Verification items for the finished model (mm, model axes). Face numbers are marked on the shaded views. A direction names the side the tool comes from. Give positions to 0.01 mm unless a question says otherwise; leave off trailing zeros. Order: outer loops, then holes, each group sorted by start corner. A loop starts at its lowest first (then second) coordinate and runs counter-clockwise, first axis right, second up. Notation, with made-up numbers: (19.5, 33) -> (61.5, 33) arc R26 cw to (61.5, 61) -> close; hole circle Ø5 at (33.5, -16). An arc over 180 degrees is marked (long way). Write each question's results on one line, items separated by ' | '. Start each with the question number.
1. Material ranges on L1, parallel to Y at x = -15, z = 28; L2, parallel to Z at x = -14, y = -24; L3, parallel to Z at x = 10, y = 3.45, recorded low to high. Write a range as from..to.
2. Cross-section at C-C, the plane y = -6. State how many separate pieces and enclosed holes the cut face has, then the cut area to 3 significant figures.
3. Mould release check, pull along Z, two halves, no side actions. Record for the marked faces 5, 6 and 7: +Z half, -Z half, draft (parallel to the pull), parting line (faces both ways), or undercut.
4. Cross-section at D-D, the plane x = -11.5. Enter the section's corners in (y, z), then the cut area to 3 significant figures.
5. Cross-section at A-A, the plane x = 10. Enter the section's corners in (y, z).
6. Cross-section at B-B, the plane z = 18. Enter the section's corners in (x, y).
7. Set-up check for the marked faces 1, 2, 3 and 4: record each of +Z, -Z, +X, -X, +Y, -Y from which the full face is reachable in a straight line by a thin tool's end or side.
8. Depth check by flat-ended pin: pin 1 Ø9 at (y, z) = (-25.5, 25.5) entering from -X; pin 2 Ø5 at (y, z) = (-24, 47) entering from +X; pin 3 Ø7 at (y, z) = (-6, 28) entering from +X; pin 4 Ø12 at (y, z) = (-23.5, 47.5) entering from -X. Enter the tip coordinate at first touch or a pass-through.
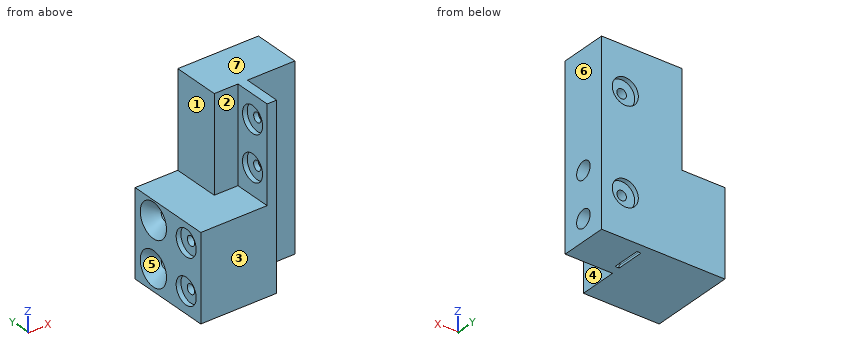
from build123d import *

# Parameters (mm, degrees)
CYLINDER007_R     = 5.5
CYLINDER007_DEPTH = 2
CYLINDER001_R     = 2
CYLINDER001_DEPTH = 32
CYLINDER006_R     = 5.5
CYLINDER006_DEPTH = 2
CYLINDER_R        = 2
CYLINDER_DEPTH    = 32
CYLINDER011_R     = 2
CYLINDER011_DEPTH = 20
CYLINDER013_R     = 5.5
CYLINDER013_DEPTH = 2
CYLINDER008_R     = 5.5
CYLINDER008_DEPTH = 2
CYLINDER002_R     = 2
CYLINDER002_DEPTH = 4
CYLINDER012_R     = 2
CYLINDER012_DEPTH = 20
CYLINDER010_R     = 5.5
CYLINDER010_DEPTH = 2
CYLINDER009_R     = 5.5
CYLINDER009_DEPTH = 2
CYLINDER003_R     = 2
CYLINDER003_DEPTH = 4
CYLINDER004_R     = 2.2
CYLINDER004_DEPTH = 22
CYLINDER015_R     = 3.7
CYLINDER015_DEPTH = 30
CYLINDER014_R     = 3.7
CYLINDER014_DEPTH = 30
CYLINDER005_R     = 2.2
CYLINDER005_DEPTH = 22
BOX002_W          = 20
BOX002_H          = 4
BOX002_DEPTH      = 76
BOX005_W          = 20
BOX005_H          = 12
BOX005_DEPTH      = 40
BOX011_W          = 18
BOX011_H          = 12
BOX011_DEPTH      = 36
BOX009_W          = 0.3
BOX009_H          = 12
BOX009_DEPTH      = 1
BOX_W             = 20
BOX_H             = 4
BOX_DEPTH         = 76
BOX012_W          = 10
BOX012_H          = 20
BOX012_DEPTH      = 40
BOX010_W          = 28
BOX010_H          = 36
BOX010_DEPTH      = 36
BOX001_W          = 4
BOX001_H          = 36
BOX001_DEPTH      = 76
CHAMFER_SIZE      = 5


with BuildPart() as cylinder007:
    # Cylinder007 → Cylinder007 (new body)
    with BuildSketch(Plane(origin=(-24, -24, 28), x_dir=(0, 0, -1), z_dir=(1, 0, 0))):
        Circle(CYLINDER007_R)
    extrude(amount=CYLINDER007_DEPTH)


with BuildPart() as fusion:
    # Cylinder001 → Cylinder001 (new body)
    with BuildSketch(Plane(origin=(-24, -24, 28), x_dir=(0, 0, -1), z_dir=(1, 0, 0))):
        Circle(CYLINDER001_R)
    extrude(amount=CYLINDER001_DEPTH)

    # Fusion: union Cylinder007
    add(cylinder007.part)


with BuildPart() as fusion_1:
    # Fusion placement: moved
    add(fusion.part.moved(Location((-8, 0, 0))))


with BuildPart() as cylinder006:
    # Cylinder006 → Cylinder006 (new body)
    with BuildSketch(Plane(origin=(-24, -24, 9), x_dir=(0, 0, -1), z_dir=(1, 0, 0))):
        Circle(CYLINDER006_R)
    extrude(amount=CYLINDER006_DEPTH)


with BuildPart() as fusion005:
    # Cylinder → Cylinder (new body)
    with BuildSketch(Plane(origin=(-24, -24, 9), x_dir=(0, 0, -1), z_dir=(1, 0, 0))):
        Circle(CYLINDER_R)
    extrude(amount=CYLINDER_DEPTH)

    # Fusion005: union Cylinder006
    add(cylinder006.part)


with BuildPart() as fusion005_1:
    # Fusion005 placement: moved
    add(fusion005.part.moved(Location((-8, 0, 0))))


with BuildPart() as cylinder011:
    # Cylinder011 → Cylinder011 (new body)
    with BuildSketch(Plane(origin=(10, 4, 58), x_dir=(1, 0, 0), z_dir=(0, -1, 0))):
        Circle(CYLINDER011_R)
    extrude(amount=CYLINDER011_DEPTH)


with BuildPart() as fusion012:
    # Cylinder013 → Cylinder013 (new body)
    with BuildSketch(Plane(origin=(10, 4, 58), x_dir=(1, 0, 0), z_dir=(0, -1, 0))):
        Circle(CYLINDER013_R)
    extrude(amount=CYLINDER013_DEPTH)

    # Fusion012: union Cylinder011
    add(cylinder011.part)


with BuildPart() as cylinder008:
    # Cylinder008 → Cylinder008 (new body)
    with BuildSketch(Plane(origin=(-4, -24, 47), x_dir=(0, 0, -1), z_dir=(1, 0, 0))):
        Circle(CYLINDER008_R)
    extrude(amount=CYLINDER008_DEPTH)


with BuildPart() as fusion007:
    # Cylinder002 → Cylinder002 (new body)
    with BuildSketch(Plane(origin=(-4, -24, 47), x_dir=(0, 0, -1), z_dir=(1, 0, 0))):
        Circle(CYLINDER002_R)
    extrude(amount=CYLINDER002_DEPTH)

    # Fusion007: union Cylinder008
    add(cylinder008.part)


with BuildPart() as cylinder012:
    # Cylinder012 → Cylinder012 (new body)
    with BuildSketch(Plane(origin=(10, 4, 18), x_dir=(1, 0, 0), z_dir=(0, -1, 0))):
        Circle(CYLINDER012_R)
    extrude(amount=CYLINDER012_DEPTH)


with BuildPart() as fusion011:
    # Cylinder010 → Cylinder010 (new body)
    with BuildSketch(Plane(origin=(10, 4, 18), x_dir=(1, 0, 0), z_dir=(0, -1, 0))):
        Circle(CYLINDER010_R)
    extrude(amount=CYLINDER010_DEPTH)

    # Fusion011: union Cylinder012
    add(cylinder012.part)


with BuildPart() as cylinder009:
    # Cylinder009 → Cylinder009 (new body)
    with BuildSketch(Plane(origin=(-4, -24, 66), x_dir=(0, 0, -1), z_dir=(1, 0, 0))):
        Circle(CYLINDER009_R)
    extrude(amount=CYLINDER009_DEPTH)


with BuildPart() as fusion006:
    # Cylinder003 → Cylinder003 (new body)
    with BuildSketch(Plane(origin=(-4, -24, 66), x_dir=(0, 0, -1), z_dir=(1, 0, 0))):
        Circle(CYLINDER003_R)
    extrude(amount=CYLINDER003_DEPTH)

    # Fusion006: union Cylinder009
    add(cylinder009.part)


with BuildPart() as cylinder004:
    # Cylinder004 → Cylinder004 (new body)
    with BuildSketch(Plane(origin=(-32, -6, 9), x_dir=(0, 0, -1), z_dir=(1, 0, 0))):
        Circle(CYLINDER004_R)
    extrude(amount=CYLINDER004_DEPTH)


with BuildPart() as fusion013:
    # Cylinder015 → Cylinder015 (new body)
    with BuildSketch(Plane(origin=(-10, -6, 9), x_dir=(0, 0, -1), z_dir=(1, 0, 0))):
        Circle(CYLINDER015_R)
    extrude(amount=CYLINDER015_DEPTH)

    # Fusion013: union Cylinder004
    add(cylinder004.part)


with BuildPart() as cylinder014:
    # Cylinder014 → Cylinder014 (new body)
    with BuildSketch(Plane(origin=(-10, -6, 28), x_dir=(0, 0, -1), z_dir=(1, 0, 0))):
        Circle(CYLINDER014_R)
    extrude(amount=CYLINDER014_DEPTH)


with BuildPart() as fusion014:
    # Cylinder005 → Cylinder005 (new body)
    with BuildSketch(Plane(origin=(-32, -6, 28), x_dir=(0, 0, -1), z_dir=(1, 0, 0))):
        Circle(CYLINDER005_R)
    extrude(amount=CYLINDER005_DEPTH)

    # Fusion014: union Cylinder014
    add(cylinder014.part)


with BuildPart() as cube002:
    # Box002 → Box002 (new body)
    with BuildSketch(Plane(origin=(0, -16, 0), x_dir=(1, 0, 0), z_dir=(0, 0, 1))):
        with Locations((10, 2)):
            Rectangle(BOX002_W, BOX002_H)
    extrude(amount=BOX002_DEPTH)


with BuildPart() as cube005:
    # Box005 → Box005 (new body)
    with BuildSketch(Plane(origin=(0, -12, 36), x_dir=(1, 0, 0), z_dir=(0, 0, 1))):
        with Locations((10, 6)):
            Rectangle(BOX005_W, BOX005_H)
    extrude(amount=BOX005_DEPTH)


with BuildPart() as cube011:
    # Box011 → Box011 (new body)
    with BuildSketch(Plane(origin=(2, -12, 0), x_dir=(1, 0, 0), z_dir=(0, 0, 1))):
        with Locations((9, 6)):
            Rectangle(BOX011_W, BOX011_H)
    extrude(amount=BOX011_DEPTH)


with BuildPart() as cube009:
    # Box009 → Box009 (new body)
    with BuildSketch(Plane(origin=(0, -12, 0), x_dir=(1, 0, 0), z_dir=(0, 0, 1))):
        with Locations((0.15, 6)):
            Rectangle(BOX009_W, BOX009_H)
    extrude(amount=BOX009_DEPTH)


with BuildPart() as cube:
    # Box → Box (new body)
    with BuildSketch(Plane.XY):
        with Locations((10, 2)):
            Rectangle(BOX_W, BOX_H)
    extrude(amount=BOX_DEPTH)


with BuildPart() as cube012:
    # Box012 → Box012 (new body)
    with BuildSketch(Plane(origin=(-14, -16, 36), x_dir=(1, 0, 0), z_dir=(0, 0, 1))):
        with Locations((5, 10)):
            Rectangle(BOX012_W, BOX012_H)
    extrude(amount=BOX012_DEPTH)


with BuildPart() as cube010:
    # Box010 → Box010 (new body)
    with BuildSketch(Plane(origin=(-32, -32, 0), x_dir=(1, 0, 0), z_dir=(0, 0, 1))):
        with Locations((14, 18)):
            Rectangle(BOX010_W, BOX010_H)
    extrude(amount=BOX010_DEPTH)


with BuildPart() as chamfer_body:
    # Box001 → Box001 (new body)
    with BuildSketch(Plane(origin=(-4, -32, 0), x_dir=(1, 0, 0), z_dir=(0, 0, 1))):
        with Locations((2, 18)):
            Rectangle(BOX001_W, BOX001_H)
    extrude(amount=BOX001_DEPTH)

    # Fusion015: union Cube002, Cube005, Cube011, Cube009, Cube, Cube012, Cube010
    add(cube002.part)
    add(cube005.part)
    add(cube011.part)
    add(cube009.part)
    add(cube.part)
    add(cube012.part)
    add(cube010.part)

    # Cut: cut Fusion014
    add(fusion014.part, mode=Mode.SUBTRACT)

    # Cut001: cut Fusion013
    add(fusion013.part, mode=Mode.SUBTRACT)

    # Cut002: cut Fusion006
    add(fusion006.part, mode=Mode.SUBTRACT)

    # Cut003: cut Fusion011
    add(fusion011.part, mode=Mode.SUBTRACT)

    # Cut004: cut Fusion007
    add(fusion007.part, mode=Mode.SUBTRACT)

    # Cut005: cut Fusion012
    add(fusion012.part, mode=Mode.SUBTRACT)

    # Cut006: cut Fusion005
    add(fusion005_1.part, mode=Mode.SUBTRACT)

    # Cut007: cut Fusion
    add(fusion_1.part, mode=Mode.SUBTRACT)

    # Chamfer
    chamfer_edges = [chamfer_body.edges().sort_by_distance(p)[0] for p in [
        (-32, -6, 11.2),
        (-32, -6, 30.2),
    ]]
    chamfer(chamfer_edges, length=CHAMFER_SIZE)


solid = chamfer_body.part
Results below:
1) L1: y = -32..-26, -22..-8.2, -3.8..4 | L2: z = 0..7, 11..26, 30..36 | L3: z = 0..12.5, 23.5..52.5, 63.5..76
2) separate pieces: 5 | enclosed holes: 2 | area: 2,480 mm²
3) face 5: undercut | face 6: draft | face 7: +Z half
4) outline: (-32, 0) -> (4, 0) -> (4, 76) -> (-16, 76) -> (-16, 36) -> (-32, 36) -> close; hole circle Ø4 at (-24, 9); hole circle Ø4 at (-24, 28); hole circle Ø4.4 at (-6, 9); hole circle Ø4.4 at (-6, 28) | area: 2,040 mm²
5) outline: (-16, 0) -> (4, 0) -> (4, 12.5) -> (2, 12.5) -> (2, 16) -> (-16, 16) -> close; (-16, 20) -> (2, 20) -> (2, 23.5) -> (4, 23.5) -> (4, 52.5) -> (2, 52.5) -> (2, 56) -> (-16, 56) -> close; (-16, 60) -> (2, 60) -> (2, 63.5) -> (4, 63.5) -> (4, 76) -> (-16, 76) -> close; hole circle Ø7.4 at (-6, 9); hole circle Ø7.4 at (-6, 28)
6) outline: (-32, -32) -> (0, -32) -> (0, -16) -> (8, -16) -> (8, 2) -> (4.5, 2) -> (4.5, 4) -> (-32, 4) -> close; (12, -16) -> (20, -16) -> (20, 4) -> (15.5, 4) -> (15.5, 2) -> (12, 2) -> close; hole (0, -12) -> (2, -12) -> (2, 0) -> (0, 0) -> close
7) face 1: +Z, -X, +Y, -Y | face 2: +Z, -X, -Y | face 3: +Z, -Z, +X, -X, -Y | face 4: +Z, -Z, +X, -Y
8) pin 1: stops at x = -32 | pin 2: stops at x = 0 | pin 3: stops at x = -10 | pin 4: stops at x = -4
